The figure shows three views and two pictorial views of one solid part (mm, origin at its lowest corner). Answer the questions. Round coordinates to 2 decimals unless told otherwise and drop trailing zeros. Write each loop counter-clockwise with the first axis right and the second up, starting at its lowest first coordinate (ties: lowest second). Pieces come first, ordered by that corner, then holes. Notation, with made-up numbers: M -3,-18 L 49,-18 A24 ccw 49,-5 Z; hole C -25,-29.75 d2. An arc over 180 degrees is marked long. Answer in a Markdown table with one row per item.
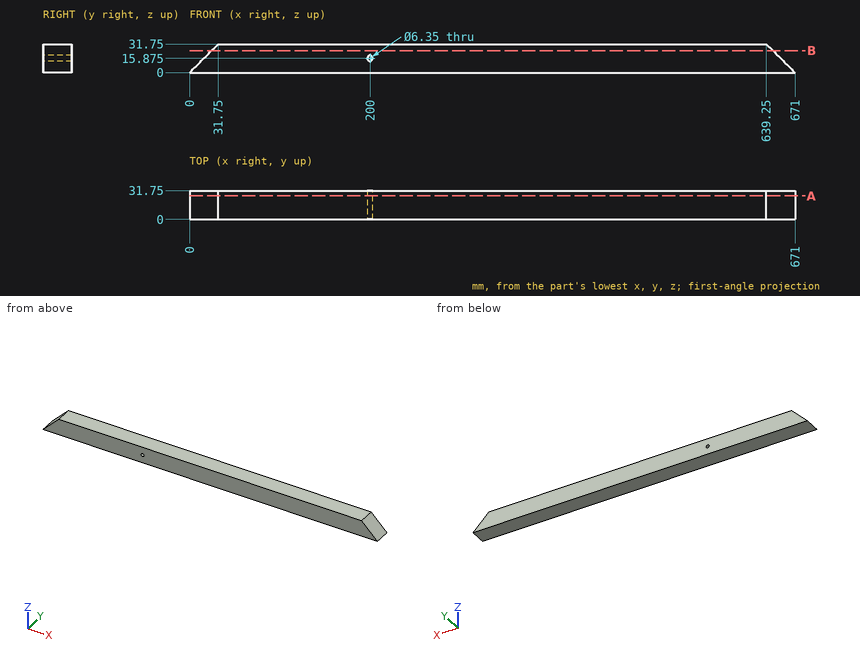
1. Given pin 1 (3 mm diameter, centred on y = 7.5, z = 6.5, fed in from -X); pin 2 (4 mm diameter, centred on y = 14, z = 15.5, fed in from -X); pin 3 (4 mm diameter, centred on y = 13.5, z = 28, fed in from -X); pin 4 (4 mm diameter, centred on x = 200, z = 15.88, fed in from +Y), each flat-ended and moving along its own axis, determine where each tip first touches the part or whether it passes through.
Calculated:
| item | result |
|---|---|
| pin 1 | stops at x = 5 |
| pin 2 | stops at x = 13.5 |
| pin 3 | stops at x = 26 |
| pin 4 | passes through |
2. The part is cut by section A-A (y = 26). Determine the outline of the cut face in (x, z) (3 decimals).
Calculated:
| item | result |
|---|---|
| outline | M 0,0 L 671,0 L 639.25,31.75 L 31.75,31.75 Z; hole C 200,15.875 d6.35 |
3. The part is cut by section B-B (z = 24.5). Determine the outline of the cut face in (x, y), plus the area to 3 significant figures.
Calculated:
| item | result |
|---|---|
| outline | M 24.5,0 L 646.5,0 L 646.5,31.75 L 24.5,31.75 Z |
| area | 19,700 mm² |
4. Consider line 1 along X through (y, z) = (22.5, 18); line 2 along X through (y, z) = (12, 14); line 3 along X through (y, z) = (17, 27). Determine where each line is inside the solid, lowest interval first. Write a range as from..to.
Calculated:
| item | result |
|---|---|
| line 1 | x = 18..197.64, 202.36..653 |
| line 2 | x = 14..197.44, 202.56..657 |
| line 3 | x = 27..644 |
